Design review of the part built by this model. Coordinates are the model's own, in mm. A direction names the side the tool comes from. Give positions to 0.01 mm unless a question says otherwise; leave off trailing zeros. Loops run counter-clockwise (first coordinate to the right, second up) from the corner with the lowest first, then second, coordinate; pieces in that order, holes last. Notation, with made-up numbers: (10.5, -32.5) - (42.5, -32.5) arc R26 ccw to (42.5, -14.5) - close; hole circle Ø8 at (77, 52). An arc over 180 degrees is marked (long way). Write each question's results on one line, items separated by ' | '.
from build123d import *

# Parameters (mm, degrees)
BOSS_EXTRUDE1_DEPTH = 28.702
SKETCH3_R           = 3.81
BOSS_EXTRUDE3_DEPTH = 78.74
BOSS_EXTRUDE4_START = 78.74
SKETCH4_R           = 3.81
BOSS_EXTRUDE4_DEPTH = 78.74


with BuildPart() as part:
    # Sketch1 → Boss-Extrude1 (new body)
    with BuildSketch(Plane(origin=(0, 0, 0), x_dir=(0, 0, -1), z_dir=(1, 0, 0))):
        with BuildLine():
            Line((1.5875, -6.148361062), (1.5875, -7.873021062))
            Line((1.5875, -7.873021062), (-1.5875, -7.873021062))
            Line((-1.5875, -7.873021062), (-1.5875, -6.148361062))
            ThreePointArc((-1.5875, -6.148361062), (0, 6.35), (1.5875, -6.148361062))
        make_face()
    extrude(amount=BOSS_EXTRUDE1_DEPTH)

    # Sketch3 → Boss-Extrude3 (add)
    with BuildSketch(Plane(origin=(28.702, 0, 0), x_dir=(0, 0, -1), z_dir=(1, 0, 0))):
        Circle(SKETCH3_R)
    extrude(amount=BOSS_EXTRUDE3_DEPTH)

    # Sketch4 → Boss-Extrude4 (add)
    with BuildSketch(Plane.ZY.offset(BOSS_EXTRUDE4_START)):
        with Locations(Location((0, 0, 0), (0, 0, 180))):
            Circle(SKETCH4_R)
    extrude(amount=-BOSS_EXTRUDE4_DEPTH)


solid = part.part
(1) Wall thickness on line 1 along X through (y, z) = (5.5, -2); line 2 along Y through (x, z) = (-52.5, -0.5): over which ranges is each line inside the solid? List them lowest first. Write a range as from..to.
Answers below:
line 1: 0..28.7 | line 2: -3.78..3.78
(2) Insertion check: P1, Ø0.9, axis at x = 8.5, y = -7.5, coming from the +Z side; P2, Ø4, axis at y = -5.5, z = -0.5, coming from the -X side; P3, Ø2, axis at y = -5.5, z = 4, coming from the -X side; P4, Ø6, axis at x = 39, y = 3, coming from the +Z side. Each pin has a flat end and moves straight along its axis. Give the tip position at first contact, or say it passes through.
Answers below:
P1: z = 1.59 | P2: x = -78.74 | P3: x = 0 | P4: z = 3.81
(3) Take a section at C-C on x = 34.5. Give the boundary of the cut face in (y, z).
Answers below:
outline: circle Ø7.62 at (0, 0)
(4) Take a section at A-A on z = 0. Give the boundary of the cut face in (x, y), plus the area to 3 significant figures.
Answers below:
outline: (-78.74, -3.81) - (0, -3.81) - (0, -7.87) - (28.7, -7.87) - (28.7, -3.81) - (107.44, -3.81) - (107.44, 3.81) - (28.7, 3.81) - (28.7, 6.35) - (0, 6.35) - (0, 3.81) - (-78.74, 3.81) - close | area: 1,610 mm2
(5) Take a section at B-B on y = 0. Give the boundary of the cut face in (x, z), plus the area to 3 significant figures.
Answers below:
outline: (-78.74, -3.81) - (0, -3.81) - (0, -6.35) - (28.7, -6.35) - (28.7, -3.81) - (107.44, -3.81) - (107.44, 3.81) - (28.7, 3.81) - (28.7, 6.35) - (0, 6.35) - (0, 3.81) - (-78.74, 3.81) - close | area: 1,560 mm2
(6) Tool access review of faces 1 (the cylindrical face through (-39.921, -3.778, 0.496)), 2 (the flat face through (14, -7.873, 0)), 3 (the flat face through (28.702, -4, 0)): name each direction out of +Z, -Z, +X, -X, +Y, -Y from which nothing blocks a thin tool from reaching the whole face with its end or side.
Answers below:
face 1: -X | face 2: +Z, -Z, +X, -X, -Y | face 3: +X
